Verification items for the finished model (mm, model axes). Give positions to 0.01 mm unless a question says otherwise; leave off trailing zeros. Write each loop counter-clockwise with the first axis right and the second up, starting at its lowest first coordinate (ties: lowest second). Pieces come first, ordered by that corner, then holes. Notation, with made-up numbers: (-12, 48.25) - (10, 48.25) arc R38 ccw to (10, 86.25) - close; hole circle Ø6 at (12, -7). An arc over 180 degrees is marked (long way). Put each result on its own line as item: value.
from build123d import *


with BuildPart() as f1:
    # F0 (on Front) → F1 (revolve)
    with BuildSketch(Plane.XZ):
        with BuildLine():
            Line((-21.984313, 0), (0, 0))
            Line((0, 0), (0, 1.25))
            Line((0, 1.25), (-10, 1.25))
            ThreePointArc((-10, 1.25), (-11.322876, 1.75), (-11.984313, 3))
            Line((-11.984313, 3), (-21.984313, 3))
            Line((-21.984313, 3), (-21.984313, 0))
        make_face()
        with BuildLine():
            Line((0, 1.25), (0, 0))
            Line((0, 0), (21.984313, 0))
            Line((21.984313, 0), (21.984313, 3))
            Line((21.984313, 3), (11.984313, 3))
            ThreePointArc((11.984313, 3), (11.322876, 1.75), (10, 1.25))
            Line((10, 1.25), (0, 1.25))
        make_face()
    revolve(axis=Axis((0, 0, 0), (1, 0, 0)))


solid = f1.part
Q1. Section check C-C, the plane x = 2.5. Record the cut outline in (y, z), plus the area to 3 significant figures.
Answers follow:
outline: circle Ø2.5 at (0, 0)
area: 4.91 mm2
Q2. Go/stop test with flat-tipped pins: pin 1 Ø2 at (x, z) = (7, -1.5) entering from -Y; pin 2 Ø3 at (x, z) = (8.5, -1) entering from +Y; pin 3 Ø1.5 at (x, z) = (11.5, 2) entering from -Y. Record where each tip stops, or that it passes through.
Answers follow:
pin 1: stops at y = -1.15
pin 2: stops at y = 1.25
pin 3: stops at y = -2.64
Q3. Section check D-D, the plane x = 13. Record the cut outline in (y, z).
Answers follow:
outline: circle Ø6 at (0, 0)
Q4. Scan lines: line 1 along Z through (x, y) = (6, 0.1); line 2 along X through (y, z) = (0.35, -2.05); line 3 along X through (y, z) = (2, -1.7). Record each from-to range of solid material in increasing order.
Answers follow:
line 1: z = -1.25 to 1.25
line 2: x = -21.98 to -11.62, 11.62 to 21.98
line 3: x = -21.98 to -11.9, 11.9 to 21.98
Q5. Section check A-A, the plane z = 0. Record the cut outline in (x, y).
Answers follow:
outline: (-21.98, -3) - (-11.98, -3) arc R2 cw to (-10, -1.25) - (10, -1.25) arc R2 cw to (11.98, -3) - (21.98, -3) - (21.98, 3) - (11.98, 3) arc R2 cw to (10, 1.25) - (-10, 1.25) arc R2 cw to (-11.98, 3) - (-21.98, 3) - close
Q6. Release check for a two-part mould opening along X. For faces 1 (the face through (-21.984, 0, 0)), 2 (the face through (17, 0, -3)), 3 (the face through (-0.14, 1.22, -0.27)), 4 (the face through (21.984, 0, 0)) record: released by +X, released by -X, zero draft, split by the parting line, or undercut.
Answers follow:
face 1: released by -X
face 2: zero draft
face 3: undercut
face 4: released by +X
